```python
from build123d import *

# Parameters (mm, degrees)
F1_DEPTH  = 10
F2_DEPTH  = 20
F3_DEPTH  = 30
F4_DEPTH  = 40
F5_DEPTH  = 50
F6_DEPTH  = 60
F7_DEPTH  = 70
F8_DEPTH  = 80
F9_DEPTH  = 90
F10_DEPTH = 100
F11_DEPTH = 106
F13_DEPTH = 200
F14_START = 62
F14_DEPTH = 60
F15_SCALE = 0.5


with BuildPart() as f1:
    # F0 (on Top) → F1 (new body)
    with BuildSketch(Plane.XY):
        with BuildLine():
            Line((36.7396253365, -84.6989331727), (33.8752285407, -94.3281765161))
            ThreePointArc((33.8752285407, -94.3281765161), (62.7668696335, -98.5786771982), (91.9348918938, -100))
            Line((91.9348918939, -100), (91.9348918939, -90))
            ThreePointArc((91.9348918938, -90), (64.2102694445, -88.6716912169), (36.7396253365, -84.6989331727))
        make_face()
        with BuildLine():
            Line((91.9348918939, -90), (91.9348918939, -100))
            ThreePointArc((91.9348918938, -100), (121.1029141542, -98.5786771982), (149.994555247, -94.3281765161))
            Line((149.994555247, -94.3281765161), (147.1301584512, -84.6989331727))
            ThreePointArc((147.1301584512, -84.6989331727), (119.6595143432, -88.6716912169), (91.9348918938, -90))
        make_face()
    extrude(amount=F1_DEPTH)

    # F0 (on Top) → F2 (join)
    with BuildSketch(Plane.XY):
        with BuildLine():
            Line((39.6049710277, -75.0664999271), (36.7396253365, -84.6989331727))
            ThreePointArc((36.7396253365, -84.6989331727), (64.2102694445, -88.6716912169), (91.9348918938, -90))
            Line((91.9348918939, -90), (91.9348918939, -80))
            ThreePointArc((91.9348918938, -80), (65.6539099829, -78.7638964963), (39.6049710277, -75.0664999271))
        make_face()
        with BuildLine():
            Line((91.9348918939, -80), (91.9348918939, -90))
            ThreePointArc((91.9348918938, -90), (119.6595143432, -88.6716912169), (147.1301584512, -84.6989331727))
            Line((147.1301584512, -84.6989331727), (144.26481276, -75.0664999271))
            ThreePointArc((144.26481276, -75.0664999271), (118.2158738048, -78.7638964963), (91.9348918938, -80))
        make_face()
    extrude(amount=F2_DEPTH)

    # F0 (on Top) → F3 (join)
    with BuildSketch(Plane.XY):
        with BuildLine():
            Line((42.4713721555, -65.4305186204), (39.6049710277, -75.0664999271))
            ThreePointArc((39.6049710277, -75.0664999271), (65.6539099829, -78.7638964963), (91.9348918938, -80))
            Line((91.9348918939, -80), (91.9348918939, -70))
            ThreePointArc((91.9348918938, -70), (67.0978231005, -68.8552026905), (42.4713721555, -65.4305186204))
        make_face()
        with BuildLine():
            Line((91.9348918939, -70), (91.9348918939, -80))
            ThreePointArc((91.9348918938, -80), (118.2158738048, -78.7638964963), (144.26481276, -75.0664999271))
            Line((144.26481276, -75.0664999271), (141.3984116322, -65.4305186204))
            ThreePointArc((141.3984116322, -65.4305186204), (116.7719606872, -68.8552026905), (91.9348918938, -70))
        make_face()
    extrude(amount=F3_DEPTH)

    # F0 (on Top) → F4 (join)
    with BuildSketch(Plane.XY):
        with BuildLine():
            Line((45.3389518797, -55.7905752255), (42.4713721555, -65.4305186204))
            ThreePointArc((42.4713721555, -65.4305186204), (67.0978231005, -68.8552026905), (91.9348918938, -70))
            Line((91.9348918939, -70), (91.9348918939, -60))
            ThreePointArc((91.9348918938, -60), (68.5420463918, -58.945505424), (45.3389518797, -55.7905752255))
        make_face()
        with BuildLine():
            Line((91.9348918939, -60), (91.9348918939, -70))
            ThreePointArc((91.9348918938, -70), (116.7719606872, -68.8552026905), (141.3984116322, -65.4305186204))
            Line((141.3984116322, -65.4305186204), (138.530831908, -55.7905752255))
            ThreePointArc((138.530831908, -55.7905752255), (115.3277373959, -58.9455054241), (91.9348918938, -60))
        make_face()
    extrude(amount=F4_DEPTH)

    # F0 (on Top) → F5 (join)
    with BuildSketch(Plane.XY):
        with BuildLine():
            Line((48.2078533621, -46.146188476), (45.3389518797, -55.7905752255))
            ThreePointArc((45.3389518797, -55.7905752255), (68.5420463918, -58.945505424), (91.9348918938, -60))
            Line((91.9348918939, -60), (91.9348918939, -50))
            ThreePointArc((91.9348918938, -50), (69.9866245248, -49.0346834469), (48.2078533621, -46.146188476))
        make_face()
        with BuildLine():
            Line((91.9348918939, -50), (91.9348918939, -60))
            ThreePointArc((91.9348918938, -60), (115.3277373959, -58.9455054241), (138.530831908, -55.7905752255))
            Line((138.530831908, -55.7905752255), (135.6619304256, -46.146188476))
            ThreePointArc((135.6619304256, -46.146188476), (113.8831592629, -49.0346834469), (91.9348918938, -50))
        make_face()
    extrude(amount=F5_DEPTH)

    # F0 (on Top) → F6 (join)
    with BuildSketch(Plane.XY):
        with BuildLine():
            Line((51.0782440128, -36.4967955891), (48.2078533621, -46.146188476))
            ThreePointArc((48.2078533621, -46.146188476), (69.9866245248, -49.0346834469), (91.9348918938, -50))
            Line((91.9348918939, -50), (91.9348918939, -40))
            ThreePointArc((91.9348918938, -40), (71.4316109538, -39.1225950652), (51.0782440128, -36.4967955891))
        make_face()
        with BuildLine():
            Line((91.9348918939, -40), (91.9348918939, -50))
            ThreePointArc((91.9348918938, -50), (113.8831592629, -49.0346834469), (135.6619304256, -46.146188476))
            Line((135.6619304256, -46.146188476), (132.7915397749, -36.4967955891))
            ThreePointArc((132.7915397749, -36.4967955891), (112.4381728339, -39.1225950652), (91.9348918938, -40))
        make_face()
    extrude(amount=F6_DEPTH)

    # F0 (on Top) → F7 (join)
    with BuildSketch(Plane.XY):
        with BuildLine():
            Line((53.9503208714, -26.8417341766), (51.0782440128, -36.4967955891))
            ThreePointArc((51.0782440128, -36.4967955891), (71.4316109538, -39.1225950652), (91.9348918938, -40))
            Line((91.9348918939, -40), (91.9348918939, -30))
            ThreePointArc((91.9348918938, -30), (72.8770701481, -29.2090736212), (53.9503208714, -26.8417341766))
        make_face()
        with BuildLine():
            Line((91.9348918939, -30), (91.9348918939, -40))
            ThreePointArc((91.9348918938, -40), (112.4381728339, -39.1225950652), (132.7915397749, -36.4967955891))
            Line((132.7915397749, -36.4967955891), (129.9194629163, -26.8417341766))
            ThreePointArc((129.9194629163, -26.8417341766), (110.9927136396, -29.2090736212), (91.9348918938, -30))
        make_face()
    extrude(amount=F7_DEPTH)

    # F0 (on Top) → F8 (join)
    with BuildSketch(Plane.XY):
        with BuildLine():
            ThreePointArc((91.9348918938, -20), (74.323080523, -19.2939217129), (56.824317494, -17.1802190931))
            Line((56.824317494, -17.1802190931), (53.9503208714, -26.8417341766))
            ThreePointArc((53.9503208714, -26.8417341766), (72.8770701481, -29.2090736212), (91.9348918938, -30))
            Line((91.9348918939, -30), (91.9348918939, -20))
        make_face()
        with BuildLine():
            ThreePointArc((127.0454662937, -17.1802190931), (109.5467032647, -19.2939217129), (91.9348918938, -20))
            Line((91.9348918939, -20), (91.9348918939, -30))
            ThreePointArc((91.9348918938, -30), (110.9927136396, -29.2090736212), (129.9194629163, -26.8417341766))
            Line((129.9194629163, -26.8417341766), (127.0454662937, -17.1802190931))
        make_face()
    extrude(amount=F8_DEPTH)

    # F0 (on Top) → F9 (join)
    with BuildSketch(Plane.XY):
        with BuildLine():
            ThreePointArc((91.9348918938, -10), (75.7697383448, -9.3769037185), (59.7005128631, -7.5113124832))
            Line((59.7005128631, -7.5113124832), (56.824317494, -17.1802190931))
            ThreePointArc((56.824317494, -17.1802190931), (74.323080523, -19.2939217129), (91.9348918938, -20))
            Line((91.9348918939, -20), (91.9348918939, -10))
        make_face()
        with BuildLine():
            ThreePointArc((124.1692709246, -7.5113124832), (108.1000454429, -9.3769037185), (91.9348918938, -10))
            Line((91.9348918939, -10), (91.9348918939, -20))
            ThreePointArc((91.9348918938, -20), (109.5467032647, -19.2939217129), (127.0454662937, -17.1802190931))
            Line((127.0454662937, -17.1802190931), (124.1692709246, -7.5113124832))
        make_face()
    extrude(amount=F9_DEPTH)

    # F0 (on Top) → F10 (join)
    with BuildSketch(Plane.XY):
        with BuildLine():
            Line((91.9348918939, 0), (61.9348918939, 0))
            Line((61.9348918939, 0), (59.7005128631, -7.5113124832))
            ThreePointArc((59.7005128631, -7.5113124832), (75.7697383448, -9.3769037185), (91.9348918938, -10))
            Line((91.9348918939, -10), (91.9348918939, 0))
        make_face()
        with BuildLine():
            Line((121.9348918939, 0), (91.9348918939, 0))
            Line((91.9348918939, 0), (91.9348918939, -10))
            ThreePointArc((91.9348918938, -10), (108.1000454429, -9.3769037185), (124.1692709246, -7.5113124832))
            Line((124.1692709246, -7.5113124832), (121.9348918939, 0))
        make_face()
    extrude(amount=F10_DEPTH)

    # F0 (on Top) → F11 (join)
    with BuildSketch(Plane.XY):
        with BuildLine():
            Line((33.7702630603, -94.3281765161), (33.8752285407, -94.3281765161))
            Line((33.8752285407, -94.3281765161), (36.7396253365, -84.6989331727))
            Line((36.7396253365, -84.6989331727), (39.6049710277, -75.0664999271))
            Line((39.6049710277, -75.0664999271), (42.4713721555, -65.4305186204))
            Line((42.4713721555, -65.4305186204), (45.3389518797, -55.7905752255))
            Line((45.3389518797, -55.7905752255), (48.2078533621, -46.146188476))
            Line((48.2078533621, -46.146188476), (51.0782440128, -36.4967955891))
            Line((51.0782440128, -36.4967955891), (53.9503208714, -26.8417341766))
            Line((53.9503208714, -26.8417341766), (56.824317494, -17.1802190931))
            Line((56.824317494, -17.1802190931), (59.7005128631, -7.5113124832))
            Line((59.7005128631, -7.5113124832), (61.9348918939, 0))
            Line((61.9348918939, 0), (51.9348918939, 0))
            Line((51.9348918939, 0), (26.696511225, -84.843869891))
            ThreePointArc((26.696511225, -84.843869891), (15.9433814137, -100.2440457927), (33.7702630603, -94.3281765161))
        make_face()
        with BuildLine():
            Line((147.1301584512, -84.6989331727), (149.994555247, -94.3281765161))
            Line((149.994555247, -94.3281765161), (150.0995207274, -94.3281765162))
            ThreePointArc((150.0995207274, -94.3281765162), (167.926402374, -100.2440457927), (157.1732725628, -84.843869891))
            Line((157.1732725628, -84.843869891), (131.9348918939, 0))
            Line((131.9348918939, 0), (121.9348918939, 0))
            Line((121.9348918939, 0), (124.1692709246, -7.5113124832))
            Line((124.1692709246, -7.5113124832), (127.0454662937, -17.1802190931))
            Line((127.0454662937, -17.1802190931), (129.9194629163, -26.8417341766))
            Line((129.9194629163, -26.8417341766), (132.7915397749, -36.4967955891))
            Line((132.7915397749, -36.4967955891), (135.6619304256, -46.146188476))
            Line((135.6619304256, -46.146188476), (138.530831908, -55.7905752255))
            Line((138.530831908, -55.7905752255), (141.3984116322, -65.4305186204))
            Line((141.3984116322, -65.4305186204), (144.26481276, -75.0664999271))
            Line((144.26481276, -75.0664999271), (147.1301584512, -84.6989331727))
        make_face()
    extrude(amount=F11_DEPTH)

    # F12 (on Right) → F13 (cut)
    with BuildSketch(Plane.YZ):
        Polygon((-84.5222696662, 31.5275415778), (-10, 106.075361371), (-105.4867506027, 106.075361371), (-105.4867506027, 31.5275415778), align=None)
    extrude(amount=F13_DEPTH, mode=Mode.SUBTRACT)

    # F12 (on Right) → F14 (cut)
    with BuildSketch(Plane.YZ.offset(F14_START)):
        Polygon((0, 79.2063996196), (-81.6366150975, 0), (0, 0), align=None)
    extrude(amount=F14_DEPTH, mode=Mode.SUBTRACT)


with BuildPart() as f1_1:
    # F15: moved
    add(f1.part.scale(F15_SCALE).moved(Location((25.9674459469, 0, 0))))


solid = f1_1.part
```
Design review of the part built by this model. Coordinates are the model's own, in mm. A direction names the side the tool comes from. Coordinates: 2 decimals unless noted, no trailing zeros. Order: outer loops, then holes, each group sorted by start corner. A loop starts at its lowest first (then second) coordinate and runs counter-clockwise, first axis right, second up. Notation, with made-up numbers: (0, 20.5) -> (53, 20.5) arc R12 cw to (53, 38.5) -> close; hole circle Ø1 at (53.25, 57.5). An arc over 180 degrees is marked (long way). One line per item, written item: value. Start each with the question number.
Q1. Insertion check: pin 1 Ø3 at (x, y) = (107, -47) entering from +Z; pin 2 Ø8.5 at (x, y) = (59.5, -45.5) entering from +Z; pin 3 Ø5 at (y, z) = (-21.5, 26.5) entering from -X. Each pin has a flat end and moves straight along its axis. Give the tip position at first contact, or say it passes through.
Q2. For probe 1 along X at (y, z) = (-24, 6.5); probe 2 along Z at (x, y) = (64.5, -47); probe 3 along X at (y, z) = (-7, 26.5), list the stretches that pass through material, from the lowest coordinate up.
Q3. Take a section at B-B, the plane y = -27. State the section outline as (x, z) points.
Q4. Take a section at C-C, the plane x = 73.5. State the section outline as (y, z) points, then the cut area to 3 significant figures.
Q5. Take a section at A-A, the plane z = 6. State the section outline as (x, y) points, then the cut area to 3 significant figures.
Q6. Take a section at D-D, the plane z = 36. State the section outline as (x, y) points, then the cut area to 3 significant figures.
Q7. Tool access review of faces 1 (the flat face through (105, -47, 15.764)), 2 (the flat face through (72, -12, 40)), 3 (the flat face through (71, -43, 0)): name each direction out of +Z, -Z, +X, -X, +Y, -Y from which nothing blocks a thin tool from reaching the whole face with its end or side.
Q8. Mouldability with a two-part tool opening along X and no side actions: class faces 4 (the flat face through (47.362, -23.736, 34.295)), 5 (the flat face through (86.967, -12, 11)), 6 (the flat face through (71.8, -20.1, 20.1)) as pulls with the +X half, pulls with the -X half, needs draft (parallel to the pull), parting line crosses it, or undercut.
Values follow:
1. pin 1: stops at z = 15.76
1. pin 2: stops at z = 10
1. pin 3: stops at x = 44.8
2. probe 1: x = 44.8 to 56.97, 86.97 to 99.07
2. probe 2: z = 0 to 5
2. probe 3: x = 49.85 to 56.97, 86.97 to 94.02
3. outline: (43.9, 0) -> (56.97, 0) -> (56.97, 13.41) -> (86.97, 13.41) -> (86.97, 0) -> (99.97, 0) -> (99.97, 31.03) -> (94.97, 31.03) -> (94.97, 25) -> (48.9, 25) -> (48.9, 31.03) -> (43.9, 31.03) -> close
4. outline: (-49.99, 0) -> (-40.82, 0) -> (0, 39.6) -> (0, 50) -> (-4.99, 50) -> (-4.99, 45) -> (-9.99, 45) -> (-9.99, 40) -> (-14.99, 40) -> (-14.99, 35) -> (-19.99, 35) -> (-19.99, 30) -> (-24.99, 30) -> (-24.99, 25) -> (-29.99, 25) -> (-29.99, 20) -> (-34.99, 20) -> (-34.99, 15) -> (-39.99, 15) -> (-39.99, 10) -> (-44.99, 10) -> (-44.99, 5) -> (-49.99, 5) -> close
4. area: 566 mm2
5. outline: (39.32, -42.42) arc R4.95 ccw (long way) to (42.85, -47.16) -> (42.91, -47.16) -> (44.34, -42.35) arc R145 ccw to (99.53, -42.35) -> (100.96, -47.16) -> (101.02, -47.16) arc R4.95 ccw (long way) to (104.55, -42.42) -> (91.93, 0) -> (86.97, 0) -> (86.97, -34.63) -> (56.97, -34.63) -> (56.97, 0) -> (51.93, 0) -> close
5. area: 1,460 mm2
6. outline: (45.38, -22.03) -> (50.38, -22.03) -> (52.94, -13.42) arc R115 ccw to (90.93, -13.42) -> (93.49, -22.03) -> (98.49, -22.03) -> (91.93, 0) -> (86.97, 0) -> (86.97, -3.71) -> (56.97, -3.71) -> (56.97, 0) -> (51.93, 0) -> close
6. area: 605 mm2
7. face 1: +Z, +X, -X, -Y
7. face 2: +Z, -Y
7. face 3: -Z, +X, -X, +Y, -Y
8. face 4: needs draft
8. face 5: undercut
8. face 6: undercut
